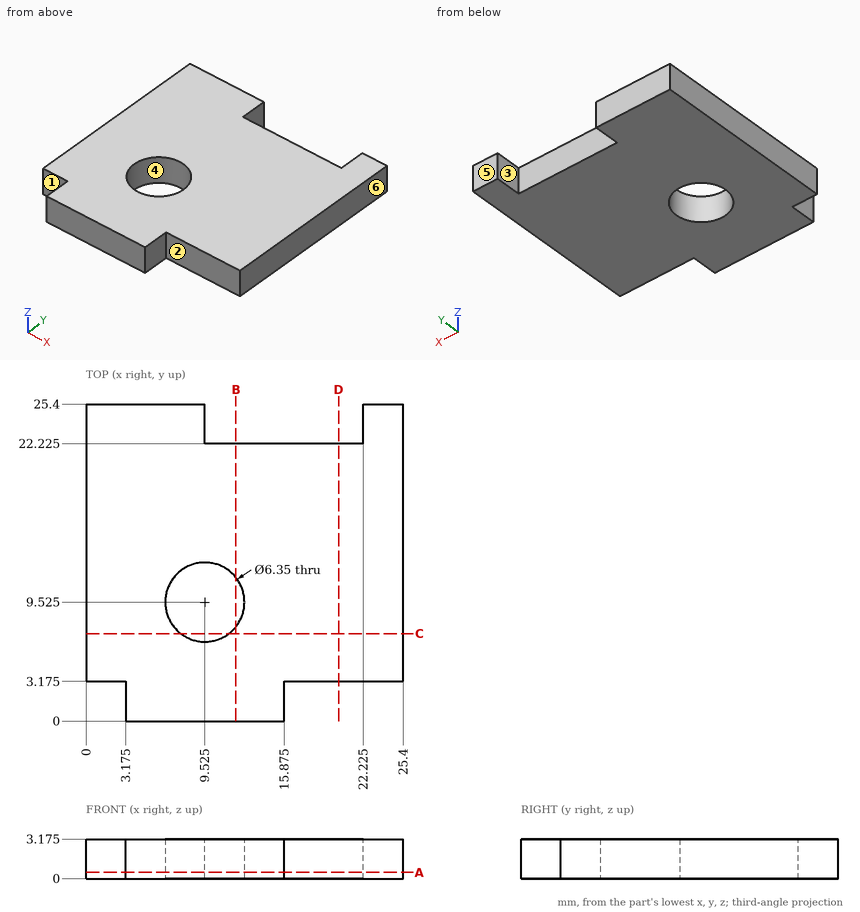
Source: three-view drawing plus pictorial views. Frame: mm from the lowest corner of the part. A direction names the side the tool comes from. Coordinates: 2 decimals unless noted, no trailing zeros. Write each loop counter-clockwise with the first axis right and the second up, starting at its lowest first coordinate (ties: lowest second). Pieces come first, ordered by that corner, then holes. Notation, with made-up numbers: (72.25, 72) - (92.25, 72) arc R32 ccw to (92.25, 98) - close; hole circle Ø9 at (-27.5, 54.5). An arc over 180 degrees is marked (long way). Return JSON: item names as keys, results as strings.
Item 1: Reachability of the marked faces 1, 2 and 3 from +Z, -Z, +X, -X, +Y, -Y: full face, straight path, thin tool, end or side. Return the list, or none.
Completed:
{"face 1": "+Z, -Z, -X, -Y", "face 2": "+Z, -Z, +X, -Y", "face 3": "+Z, -Z, +Y"}
Item 2: Section query D-D (x = 20.25). Output: boundary loops of the cut face in (y, z) (3 decimals).
Completed:
{"outline": "(3.175, 0) - (22.225, 0) - (22.225, 3.175) - (3.175, 3.175) - close"}
Item 3: Line query: L1, parallel to X at y = 9.5, z = 0.7; L2, parallel to Y at x = 17, z = 1.5 (3 decimals); L3, parallel to Y at x = 2, z = 2.2 (3 decimals). Output: solid intervals per line, ascending.
Completed:
{"L1": "x = 0 to 6.35, 12.7 to 25.4", "L2": "y = 3.175 to 22.225", "L3": "y = 3.175 to 25.4"}
Item 4: Section query A-A (z = 0.5). Output: boundary loops of the cut face in (x, y) (3 decimals).
Completed:
{"outline": "(0, 3.175) - (3.175, 3.175) - (3.175, 0) - (15.875, 0) - (15.875, 3.175) - (25.4, 3.175) - (25.4, 25.4) - (22.225, 25.4) - (22.225, 22.225) - (9.525, 22.225) - (9.525, 25.4) - (0, 25.4) - close; hole circle Ø6.35 at (9.525, 9.525)"}
Item 5: Section query B-B (x = 12). Output: boundary loops of the cut face in (y, z) (3 decimals).
Completed:
{"outline": "(0, 0) - (7.536, 0) - (7.536, 3.175) - (0, 3.175) - close; (11.514, 0) - (22.225, 0) - (22.225, 3.175) - (11.514, 3.175) - close"}
Item 6: Pull-direction query (Y, two-part tool) for the marked faces 4, 5 and 6; classes: +Y half, -Y half, draft (parallel to the pull), parting line (faces both ways), or undercut.
Completed:
{"face 4": "undercut", "face 5": "+Y half", "face 6": "draft"}
Item 7: Pin query (flat end, axial travel): pin 1 Ø1.6 at (y, z) = (2, 2) entering from -X (3 decimals); pin 2 Ø5.5 at (x, y) = (9.525, 9.525) entering from +Z; pin 3 Ø1 at (x, z) = (1.5, 2) entering from -Y (3 decimals); pin 4 Ø1.6 at (x, z) = (18, 2) entering from +Y (3 decimals). Return the tip coordinate at first contact, or that it passes through.
Completed:
{"pin 1": "stops at x = 3.175", "pin 2": "passes through", "pin 3": "stops at y = 3.175", "pin 4": "stops at y = 22.225"}
Item 8: Section query C-C (y = 7). Output: boundary loops of the cut face in (x, z) (3 decimals).
Completed:
{"outline": "(0, 0) - (7.6, 0) - (7.6, 3.175) - (0, 3.175) - close; (11.45, 0) - (25.4, 0) - (25.4, 3.175) - (11.45, 3.175) - close"}
